Can you work these out from the model? Positions are in its coordinate system, mm. A direction names the side the tool comes from. Give positions to 0.01 mm unless a question says otherwise; leave off trailing zeros. Loops run counter-clockwise (first coordinate to the right, second up) from the corner with the lowest first, then second, coordinate; pieces in that order, holes last.
from build123d import *

# Parameters (mm, degrees)
SKETCH_1_R             = 1.5
EXTRUDE_1_DEPTH        = 2
SKETCH_2_W             = 16.5
SKETCH_2_H             = 7
EXTRUDE_2_DEPTH        = 6
SKETCH_3_W             = 6
SKETCH_3_H             = 10
EXTRUDE_3_DEPTH        = 10
PATTERN_LINEAR_1_COUNT = 2
PATTERN_LINEAR_1_PITCH = 15
PATTERN_LINEAR_2_COUNT = 2
PATTERN_LINEAR_2_PITCH = 15
SKETCH_4_W             = 14.5
SKETCH_4_H             = 4
CUT_EXTRUDE_1_DEPTH    = 5


with BuildPart() as part:
    # 草图1 → 凸台-拉伸1 (new body)
    with BuildSketch(Plane(origin=(0, 0, 0), x_dir=(1, 0, 0), z_dir=(0, 1, 0))):
        Polygon((-20, 15), (20, 15), (20, 2), (8.25, -10), (8.25, -15), (-8.25, -15), (-8.25, -10), (-20, 2), align=None)
        with Locations(Location((-10, -4, 0), (0, 0, 270))):
            Circle(SKETCH_1_R, mode=Mode.SUBTRACT)
        with Locations(Location((10, -4, 0), (0, 0, 270))):
            Circle(SKETCH_1_R, mode=Mode.SUBTRACT)
    extrude(amount=EXTRUDE_1_DEPTH)

    # 草图2 → 凸台-拉伸2 (add)
    with BuildSketch(Plane(origin=(0, 2, 0), x_dir=(1, 0, 0), z_dir=(0, 1, 0))):
        with Locations((0, -11.5)):
            Rectangle(SKETCH_2_W, SKETCH_2_H)
    extrude(amount=EXTRUDE_2_DEPTH)

    # 草图3 → 凸台-拉伸3 (add)
    with BuildSketch(Plane.XZ):
        with Locations((0, -8)):
            Rectangle(SKETCH_3_W, SKETCH_3_H)
    extrude_3 = extrude(amount=EXTRUDE_3_DEPTH)

    # 阵列(线性)1: 凸台-拉伸3 ×2
    with Locations(*[(i * PATTERN_LINEAR_1_PITCH, 0, 0) for i in range(1, PATTERN_LINEAR_1_COUNT)]):
        add(extrude_3)

    # 阵列(线性)2: 凸台-拉伸3 ×2
    with Locations(*[(-i * PATTERN_LINEAR_2_PITCH, 0, 0) for i in range(1, PATTERN_LINEAR_2_COUNT)]):
        add(extrude_3)

    # 草图4 → 切除-拉伸1 (cut)
    with BuildSketch(Plane.XY.offset(15)):
        with Locations((0, 5)):
            Rectangle(SKETCH_4_W, SKETCH_4_H)
    extrude(amount=-CUT_EXTRUDE_1_DEPTH, mode=Mode.SUBTRACT)


solid = part.part
(1) Thinking about a two-plate mould opening in Y: for faces 4 (the flat face through (0, 8, 11)), 5 (the flat face through (0, 7, 13)), 6 (the flat face through (-15, -5, -13)), which applies, pulls with the +Y half, pulls with the -Y half, needs draft (parallel to the pull), parting line crosses it, or undercut?
Returned:
face 4: pulls with the +Y half
face 5: undercut
face 6: needs draft
(2) Suppose I cut it at A-A on y = -3. List the corners of the cut face in (x, z) for me, plus the area to 3 significant figures.
Returned:
outline: (-18, -13) - (-12, -13) - (-12, -3) - (-18, -3) - close; (-3, -13) - (3, -13) - (3, -3) - (-3, -3) - close; (12, -13) - (18, -13) - (18, -3) - (12, -3) - close
area: 180 mm2
(3) Suppose I cut it at C-C on y = 1.25. List the corners of the cut face in (x, z) for me.
Returned:
outline: (-20, -15) - (20, -15) - (20, -2) - (8.25, 10) - (8.25, 15) - (-8.25, 15) - (-8.25, 10) - (-20, -2) - close; hole circle Ø3 at (-10, 4); hole circle Ø3 at (10, 4)
(4) Please list where these lines run through material, in increasing order: probe 1 along Y at (x, z) = (4, 13.5); probe 2 along X at (y, z) = (-4.5, -8.25); probe 3 along X at (y, z) = (0.5, 4) (3 decimals).
Returned:
probe 1: y = 0 to 3, 7 to 8
probe 2: x = -18 to -12, -3 to 3, 12 to 18
probe 3: x = -14.125 to -11.5, -8.5 to 8.5, 11.5 to 14.125
(5) Will these pins go through, and if not, where does the flat tip stop? P1, Ø1.8, axis at x = 16.5, y = -5.5, coming from the +Z side; P2, Ø3, axis at y = 1.5, z = 1, coming from the +X side; P3, Ø1.5, axis at x = 2, z = 12.5, coming from the -Y side.
Returned:
P1: stops at z = -3
P2: stops at x = 18.53
P3: stops at y = 0
(6) Suppose I cut it at D-D on x = 10. List the corners of the cut face in (y, z) for me.
Returned:
outline: (0, -15) - (2, -15) - (2, 2.5) - (0, 2.5) - close; (0, 5.5) - (2, 5.5) - (2, 8.21) - (0, 8.21) - close
(7) Which directions (+Z, -Z, +X, -X, +Y, -Y) give clear straight access to the entire face, cutting with the end or side of a thin tool? Please do faces 1 (the flat face through (3, -5, -8)), 2 (the flat face through (0, -5, -13)), 3 (the flat face through (-15, -5, -3)).
Returned:
face 1: +Z, -Z, -Y
face 2: -Z, +X, -X, -Y
face 3: +Z, +X, -X, -Y
(8) Suppose I cut it at B-B on z = 4. List the corners of the cut face in (x, y) for me (3 decimals), plus the area to 3 significant figures.
Returned:
outline: (-14.125, 0) - (-11.5, 0) - (-11.5, 2) - (-14.125, 2) - close; (-8.5, 0) - (8.5, 0) - (8.5, 2) - (-8.5, 2) - close; (11.5, 0) - (14.125, 0) - (14.125, 2) - (11.5, 2) - close
area: 44.5 mm2
